Autodesk Inventor part; units mm, degrees
ref_plane "YZ Plane" through (0, 0, 0) normal (1, 0, 0) x (0, 1, 0)
ref_plane "XZ Plane" through (0, 0, 0) normal (0, 1, 0) x (-1, 0, 0)
ref_plane "XY Plane" through (0, 0, 0) normal (0, 0, 1) x (1, 0, 0)
sketch "Sketch1" plane through (0, 0, 0) normal (0, 1, 0) x (-1, 0, 0)
  line L0 (107.95, -174.625) -> (-107.95, -174.625)
  line L1 (-107.95, -174.625) -> (-107.95, 174.625)
  line L2 (-107.95, 174.625) -> (107.95, 174.625)
  line L3 (107.95, 174.625) -> (107.95, -174.625)
  line L4 (107.95, -174.625) -> (-107.95, 174.625) construction
  line L5 (-107.95, -174.625) -> (107.95, 174.625) construction
  point P0 (0, 0)
  dimension "d0" = 215.9
  dimension "d1" = 349.25
extrude "Thickness" add sketch "Sketch1" along normal blind 3.175
sketch "Cutout Sketch" plane through (0, 3.175, 0) normal (0, 1, 0) x (1, 0, 0)
  line L0 (107.95, -174.625) -> (107.95, 174.625)
  line L1 (107.95, 174.625) -> (-107.95, 174.625)
  line L2 (-107.95, 174.625) -> (-107.95, -174.625)
  line L3 (-107.95, -174.625) -> (107.95, -174.625)
  line L4 (-82.55, 136.525) -> (82.55, 136.525)
  line L5 (82.55, 136.525) -> (82.55, -136.525)
  line L6 (82.55, -136.525) -> (-82.55, -136.525)
  line L7 (-82.55, -136.525) -> (-82.55, 136.525)
  point P0 (0, 0)
  dimension "d4" = 25.4
  dimension "d5" = 38.1
  dimension "d8" = 38.1
  dimension "d9" = 25.4
extrude "Cutout" cut sketch "Cutout Sketch" against normal blind 25.4 contours L4 L5 L6 L7
sketch "Sketch3" plane through (0, 3.175, 0) normal (0, 1, 0) x (1, 0, 0)
  line L0 (44.45, 149.225) -> (44.45, 137.9537)
  line L1 (44.45, 137.9537) -> (49.1744, 137.9537)
  line L2 (49.1744, 137.9537) -> (49.1744, 136.525)
  line L3 (49.1744, 136.525) -> (54.737, 136.525)
  line L4 (54.737, 136.525) -> (54.737, 137.9537)
  line L5 (54.737, 137.9537) -> (59.563, 137.9537)
  line L6 (59.563, 137.9537) -> (59.563, 136.525)
  line L7 (59.563, 136.525) -> (65.1256, 136.525)
  line L8 (65.1256, 136.525) -> (65.1256, 137.9537)
  line L9 (65.1256, 137.9537) -> (69.85, 137.9537)
  line L10 (69.85, 149.225) -> (69.85, 137.9537)
  line L11 (44.45, 149.225) -> (69.85, 149.225)
  circle A0 centre (65.0875, 144.0656) radius 2.0955
  circle A1 centre (49.2125, 144.0656) radius 2.0955
  line L12 (-69.85, 149.225) -> (-69.85, 137.9537)
  line L13 (-69.85, 137.9537) -> (-65.1256, 137.9537)
  line L14 (-65.1256, 137.9537) -> (-65.1256, 136.525)
  line L15 (-65.1256, 136.525) -> (-59.563, 136.525)
  line L16 (-59.563, 136.525) -> (-59.563, 137.9537)
  line L17 (-59.563, 137.9537) -> (-54.737, 137.9537)
  line L18 (-54.737, 137.9537) -> (-54.737, 136.525)
  line L19 (-54.737, 136.525) -> (-49.1744, 136.525)
  line L20 (-49.1744, 136.525) -> (-49.1744, 137.9537)
  line L21 (-49.1744, 137.9537) -> (-44.45, 137.9537)
  line L22 (-44.45, 149.225) -> (-44.45, 137.9537)
  line L23 (-69.85, 149.225) -> (-44.45, 149.225)
  circle A2 centre (-49.2125, 144.0656) radius 2.0955
  circle A3 centre (-65.0875, 144.0656) radius 2.0955
  point P0 (0, 0)
hole "Hole1" at (65.0875, 3.175, -144.0656) at (49.2125, 3.175, -144.0656) at (-65.0875, 3.175, -144.0656) at (-49.2125, 3.175, -144.0656) direction (0, -1, 0) diameter 3.5 depth 2
sketch "Sketch4" plane through (0, 3.175, 0) normal (0, 1, 0) x (1, 0, 0)
  circle A0 centre (-65.0875, 144.0656) radius 1.75
  circle A1 centre (65.0875, 144.0656) radius 1.75
  circle A2 centre (49.2125, 144.0656) radius 1.75
  circle A3 centre (-49.2125, 144.0656) radius 1.75
  line L0 (-82.55, 136.525) -> (82.55, 136.525)
  line L1 (82.55, 136.525) -> (82.55, -136.525)
  line L2 (82.55, -136.525) -> (-82.55, -136.525)
  line L3 (-82.55, -136.525) -> (-82.55, 136.525)
  line L4 (107.95, 174.625) -> (-107.95, 174.625)
  line L5 (-107.95, 174.625) -> (-107.95, -174.625)
  line L6 (-107.95, -174.625) -> (107.95, -174.625)
  line L7 (107.95, -174.625) -> (107.95, 174.625)
  point P0 (0, 0)
  point P1 (-95.25, -161.925)
  point P2 (-95.25, 161.925)
  point P3 (95.25, -161.925)
  point P4 (95.25, 161.925)
  point P5 (95.25, -53.975)
  point P6 (95.25, 53.975)
  point P7 (0, -161.925)
  point P8 (0, 161.925)
  point P9 (-95.25, -53.975)
  point P10 (-95.25, 53.975)
  point P11 (0, -136.525)
  point P12 (0, 136.525)
  dimension "d17" = 12.7
  dimension "d18" = 12.7
  dimension "d19" = 12.7
  dimension "d20" = 323.85
  dimension "d21" = 107.95
  dimension "d22" = 107.95
  dimension "d23" = 12.7
hole "Hole2" at (-95.25, 3.175, 161.925) at (-95.25, 3.175, -161.925) at (95.25, 3.175, 161.925) at (95.25, 3.175, -161.925) at (95.25, 3.175, 53.975) at (95.25, 3.175, -53.975) at (0, 3.175, 161.925) at (0, 3.175, -161.925) at (-95.25, 3.175, 53.975) at (-95.25, 3.175, -53.975) direction (0, -1, 0) diameter 3.5 end through all
properties part number "NASA-20-EBOX-T2-01" material "Polycarbonate, Clear"
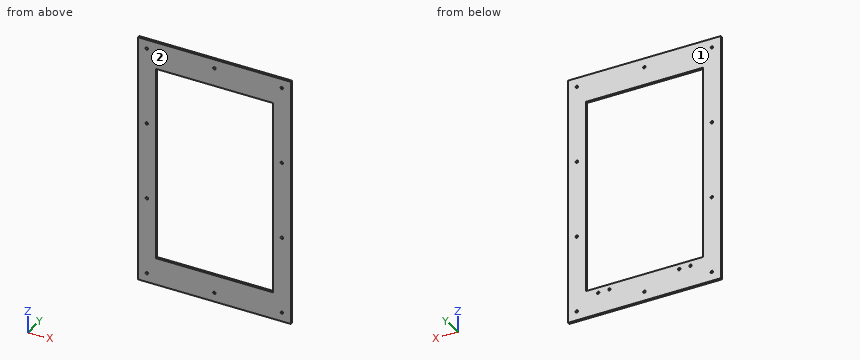
Can you work these out from the model? Positions are in its coordinate system, mm. Face numbers are marked on the shaded views. Coordinates: 2 decimals unless noted, no trailing zeros. Order: outer loops, then holes, each group sorted by start corner. A loop starts at its lowest first (then second) coordinate and runs counter-clockwise, first axis right, second up. Notation, with made-up numbers: M -3.5,-8.5 L 48.5,-8.5 A16 cw 48.5,5.5 Z; hole C 40.5,26 d1. An arc over 180 degrees is marked long. Write item = value, one per line.
(1) Suppose I cut it at C-C on z = -31.5. Please give me the cut outline in (x, y) (3 decimals).
Results are:
outline = M -107.95,0 L -82.55,0 L -82.55,3.175 L -107.95,3.175 Z; M 82.55,0 L 107.95,0 L 107.95,3.175 L 82.55,3.175 Z
(2) If we mould it in two halves opening along Y, with no side actions, what happens to the marked faces 1 and 2? For each: pulls with the +Y half, pulls with the -Y half, needs draft (parallel to the pull), parting line crosses it, or undercut.
Results are:
face_1 = pulls with the +Y half
face_2 = pulls with the -Y half
(3) Suppose I cut it at B-B on x = 14.5. Please give me the cut outline in (y, z) (3 decimals), plus the area to 3 significant figures.
Results are:
outline = M 0,-174.625 L 3.175,-174.625 L 3.175,-136.525 L 0,-136.525 Z; M 0,136.525 L 3.175,136.525 L 3.175,174.625 L 0,174.625 Z
area = 242 mm2
(4) I need wall thicknesses on line 1 along Z through (x, y) = (95.25, 1.7) (3 decimals); line 2 along X through (y, z) = (1.45, -46.5); line 3 along Z through (x, y) = (-20, 2.25) (3 decimals). Which ranges of each line are inside material? Lowest first, please. Write a range as [from, to].
Results are:
line_1 = [-174.625, -163.675], [-160.175, -55.725], [-52.225, 52.225], [55.725, 160.175], [163.675, 174.625]
line_2 = [-107.95, -82.55], [82.55, 107.95]
line_3 = [-174.625, -136.525], [136.525, 174.625]
(5) Suppose I cut it at A-A on y = 0.6. State how many separate pieces and enclosed holes the cut face has, plus the area to 3 significant figures.
Results are:
separate_pieces = 1
enclosed_holes = 11
area = 30,200 mm2
(6) For pin 1 Ø3 at (x, z) = (-65.09, -144.07) entering from +Y (3 decimals); pin 2 Ø3 at (x, z) = (65.5, -144) entering from +Y (3 decimals), each with a flat end and sliding along its axis, tell me the tip position at first contact or that it passes through.
Results are:
pin_1 = 1.175
pin_2 = 3.175
